Could you check a few things on this model? Use its own coordinates, in mm. Round coordinates to 2 decimals unless told otherwise and drop trailing zeros. Write each loop counter-clockwise with the first axis right and the second up, starting at its lowest first coordinate (ties: lowest second). Pieces come first, ordered by that corner, then holes. Notation, with made-up numbers: (24, 47.25) -> (73, 47.25) arc R31 ccw to (73, 86.25) -> close; hole circle Ø11 at (6, 38.25). An arc over 180 degrees is marked (long way). Answer as CSV lines item,"result". Start each with the question number.
Q1. Will this pin go through, and if not, where does the flat tip stop? pin 1 Ø5 at (x, y) = (19.22, 90) entering from -Z.
Q2. Imagine slicing it at A-A on y = 90. Please give me the cut outline in (x, z).
Q3. If I drill on line 1 (X direction, y = 90.5, z = 6.5); line 2 (Y direction, x = 21.5, z = 7.5); line 3 (Y direction, x = -78, z = 0.5), over which ranges is the centre line in solid material (lowest first)? Write a range as [from, to].
Q4. Imagine slicing it at B-B on y = 30. Please give me the cut outline in (x, z).
from build123d import *

# Parameters (mm, degrees)
ESQUISSE1_W             = 300
ESQUISSE1_H             = 100
BOSS_EXTRU_1_DEPTH      = 10
ESQUISSE2_R             = 3
ENL_V_MAT_EXTRU_1_DEPTH = 212.887970305
ESQUISSE3_R             = 5
ENL_V_MAT_EXTRU_2_DEPTH = 212.887970305


with BuildPart() as part:
    # Esquisse1 → Boss.-Extru.1 (new body)
    with BuildSketch(Plane.XY):
        with Locations((36.538231899, 50)):
            Rectangle(ESQUISSE1_W, ESQUISSE1_H)
    extrude(amount=BOSS_EXTRU_1_DEPTH)

    # Esquisse2 → Enlèv. mat.-Extru.1 (cut, through all)
    with BuildSketch(Plane.XY.offset(10)):
        with Locations((49.22419633, 90)):
            Circle(ESQUISSE2_R)
        with Locations((19.22419633, 90)):
            Circle(ESQUISSE2_R)
    extrude(amount=-ENL_V_MAT_EXTRU_1_DEPTH, mode=Mode.SUBTRACT)

    # Esquisse3 → Enlèv. mat.-Extru.2 (cut, through all)
    with BuildSketch(Plane.XY.offset(10)):
        with Locations((-73.461768101, 30)):
            Circle(ESQUISSE3_R)
        with Locations((146.538231899, 30)):
            Circle(ESQUISSE3_R)
    extrude(amount=-ENL_V_MAT_EXTRU_2_DEPTH, mode=Mode.SUBTRACT)


solid = part.part
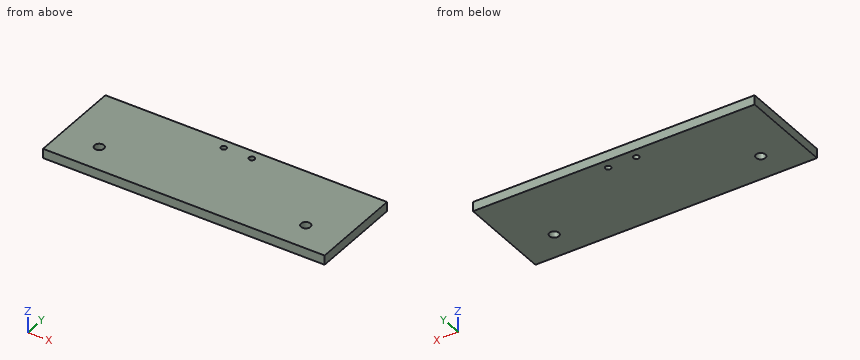
Checks:
1,pin 1,"through"
2,outline,"(-113.46, 0) -> (16.22, 0) -> (16.22, 10) -> (-113.46, 10) -> close; (22.22, 0) -> (46.22, 0) -> (46.22, 10) -> (22.22, 10) -> close; (52.22, 0) -> (186.54, 0) -> (186.54, 10) -> (52.22, 10) -> close"
3,line 1,"[-113.46, 16.27], [22.18, 46.27], [52.18, 186.54]"
3,line 2,"[0, 88.05], [91.95, 100]"
3,line 3,"[0, 27.9], [32.1, 100]"
4,outline,"(-113.46, 0) -> (-78.46, 0) -> (-78.46, 10) -> (-113.46, 10) -> close; (-68.46, 0) -> (141.54, 0) -> (141.54, 10) -> (-68.46, 10) -> close; (151.54, 0) -> (186.54, 0) -> (186.54, 10) -> (151.54, 10) -> close"
